```python
from build123d import *

# Parameters (mm, degrees)
F1_W        = 101.6
F1_H        = 101.6
F1_W_2      = 96.52
F1_H_2      = 96.52
F2_DEPTH    = 2.54
F3_T1_DEPTH = 123.5970452561
F3_T3_DEPTH = 123.5970452561
F4_DEPTH    = 2.54


# Not quite as in the source:
# - a fillet or chamfer that OpenCascade refuses, or shapes differently, is made with other operations: its cross-section is extruded or revolved along the edge and cut away or added


with BuildPart() as f2:
    # F1 (on offset) → F2 (new body)
    with BuildSketch(Plane.XY.offset(101.6)):
        with Locations((-130.4673959928, -63.7241914409)):
            Rectangle(F1_W, F1_H)
        with Locations((-130.4673959928, -63.7241914409)):
            Rectangle(F1_W_2, F1_H_2, mode=Mode.SUBTRACT)
        with Locations((-130.4673959928, -63.7241914409)):
            Rectangle(F1_W_2, F1_H_2)
    extrude(amount=F2_DEPTH)

    # F3: fillet of radius 5.08 on 4 edges, made by hand

    # F3_s2 → F3_t1 (cut)
    with BuildSketch(Plane.YZ.offset(-192.2659186209)):
        with BuildLine():
            ThreePointArc((-114.5241914409, 101.6), (-112.6647823896, 103.4594090512), (-110.1247823896, 104.14))
            Line((-110.1247823896, 104.14), (-114.5241914409, 104.14))
            Line((-114.5241914409, 104.14), (-114.5241914409, 101.6))
        make_face()
        with BuildLine():
            ThreePointArc((-12.9241914409, 101.6), (-14.7836004921, 103.4594090512), (-17.3236004921, 104.14))
            Line((-17.3236004921, 104.14), (-12.9241914409, 104.14))
            Line((-12.9241914409, 104.14), (-12.9241914409, 101.6))
        make_face()
    extrude(amount=F3_T1_DEPTH, mode=Mode.SUBTRACT)

    # F3_s4 → F3_t3 (cut)
    with BuildSketch(Plane.XZ.offset(1.9256688128)):
        with BuildLine():
            ThreePointArc((-79.6673959928, 101.6), (-81.526805044, 103.4594090512), (-84.066805044, 104.14))
            Line((-84.066805044, 104.14), (-79.6673959928, 104.14))
            Line((-79.6673959928, 104.14), (-79.6673959928, 101.6))
        make_face()
        with BuildLine():
            ThreePointArc((-181.2673959928, 101.6), (-179.4079869416, 103.4594090512), (-176.8679869416, 104.14))
            Line((-176.8679869416, 104.14), (-181.2673959928, 104.14))
            Line((-181.2673959928, 104.14), (-181.2673959928, 101.6))
        make_face()
    extrude(amount=F3_T3_DEPTH, mode=Mode.SUBTRACT)

    # F1 (on offset) → F4 (join)
    with BuildSketch(Plane.XY.offset(101.6)):
        with Locations((-130.4673959928, -63.7241914409)):
            Rectangle(F1_W_2, F1_H_2)
    extrude(amount=-F4_DEPTH)


solid = f2.part
```
CAD build for the part. Positions are in the model's coordinates, mm. A direction names the side the tool comes from. Coordinates: 2 decimals unless noted, no trailing zeros. Loops run counter-clockwise (first coordinate to the right, second up) from the corner with the lowest first, then second, coordinate; pieces in that order, holes last. Notation, with made-up numbers: (6.5, -31.75) - (48.5, -31.75) arc R23 cw to (48.5, -6.75) - close; hole circle Ø11 at (-0.5, 5.25). An arc over 180 degrees is marked (long way). Return JSON: item names as keys, results as strings.
1. Band-saw the part on B-B (x = -170). Give the cut face in (y, z).
Result:
{"outline": "(-114.52, 101.6) - (-111.98, 101.6) - (-111.98, 99.06) - (-15.46, 99.06) - (-15.46, 101.6) - (-12.92, 101.6) arc R5.08 ccw to (-17.32, 104.14) - (-110.12, 104.14) arc R5.08 ccw to start"}
2. Drop flat-ended pins along their axis: pin 1 (0.8 mm diameter, centred on y = -78.5, z = 100.5, fed in from +X); pin 2 (0.8 mm diameter, centred on x = -134, z = 101, fed in from -Y); pin 3 (0.8 mm diameter, centred on x = -140, z = 100, fed in from +Y). Give the stop position or say it passes through.
Result:
{"pin 1": "stops at x = -82.21", "pin 2": "stops at y = -111.98", "pin 3": "stops at y = -15.46"}
3. Band-saw the part on C-C (z = 100.1). Give the cut face in (x, y).
Result:
{"outline": "(-178.73, -111.98) - (-82.21, -111.98) - (-82.21, -15.46) - (-178.73, -15.46) - close"}
4. 3-axis set-ups, long thin cutter, end or side, ignore diameter. For faces 1 (the flat face through (-131, -15.464, 100)), 2 (the flat face through (-178.727, -64, 100)), 3 (the flat face through (-82.207, -64, 100)), 4 (the flat face through (-131, -111.984, 100)): which of +Z, -Z, +X, -X, +Y, -Y reach the whole face in a straight line?
Result:
{"face 1": "-Z, +X, -X, +Y", "face 2": "-Z, -X, +Y, -Y", "face 3": "-Z, +X, +Y, -Y", "face 4": "-Z, +X, -X, -Y"}
5. Band-saw the part on A-A (y = -56). Give the cut face in (x, z).
Result:
{"outline": "(-181.27, 101.6) - (-178.73, 101.6) - (-178.73, 99.06) - (-82.21, 99.06) - (-82.21, 101.6) - (-79.67, 101.6) arc R5.08 ccw to (-84.07, 104.14) - (-176.87, 104.14) arc R5.08 ccw to start"}
6. Probe L1, parallel to Y at x = -153, z = 101.45; L2, parallel to X at y = -90, z = 99.6; L3, parallel to X at y = -73, z = 102.6. List the from-to ranges inside material, lowest first. Write a range as from..to.
Result:
{"L1": "y = -111.98..-15.46", "L2": "x = -178.73..-82.21", "L3": "x = -180.51..-80.42"}
